Read the model definition and answer for the solid it produces. Units are mm, in the model's axes. A direction names the side the tool comes from. Give positions to 0.01 mm unless a question says otherwise; leave off trailing zeros. Write each loop counter-clockwise with the first axis right and the second up, starting at its lowest first coordinate (ties: lowest second). Pieces come first, ordered by that corner, then holes. Notation, with made-up numbers: (18, 11) -> (36, 11) arc R33 ccw to (36, 48) -> close; hole circle Ø2 at (-12.5, 84). An arc over 180 degrees is marked (long way). Put each result on its own line as item: value. Start each with the question number.
from build123d import *

# Parameters (mm, degrees)
F0_R     = 14.2875
F1_DEPTH = 25.4
F2_DEPTH = 25.4
F3_DEPTH = 50.8


with BuildPart() as f1:
    # F0 (on Front) → F1 (new body)
    with BuildSketch(Plane.XZ):
        with BuildLine():
            ThreePointArc((5.2887591577, -28.0813043068), (21.9961009946, -18.240125165), (28.575, 0))
            ThreePointArc((28.575, 0), (22.118144808, 18.0919400633), (5.6655830094, 28.0077095487))
            ThreePointArc((5.6655830094, 28.0077095487), (-28.5743551441, 0.1919716148), (5.2887591577, -28.0813043068))
        make_face()
        with BuildLine():
            ThreePointArc((-13.4703841816, 4.7625), (0, 14.2875), (13.4703841816, 4.7625))
            Line((13.4703841816, 4.7625), (22.225, 4.7625))
            Line((22.225, 4.7625), (22.225, -4.7625))
            Line((22.225, -4.7625), (13.4703841816, -4.7625))
            ThreePointArc((13.4703841816, -4.7625), (0, -14.2875), (-13.4703841816, -4.7625))
            Line((-13.4703841816, -4.7625), (-22.225, -4.7625))
            Line((-22.225, -4.7625), (-22.225, 4.7625))
            Line((-22.225, 4.7625), (-13.4703841816, 4.7625))
        make_face(mode=Mode.SUBTRACT)
        with BuildLine():
            ThreePointArc((73.025, 0), (66.3713381906, 14.464898875), (51.0582494002, 18.8253835536))
            ThreePointArc((51.0582494002, 18.8253835536), (34.9584276531, -1.1280408576), (53.304272269, -19.0381885775))
            ThreePointArc((53.304272269, -19.0381885775), (67.2061212058, -13.7054708652), (73.025, 0))
        make_face()
        with Locations((53.975, 0)):
            Circle(F0_R, mode=Mode.SUBTRACT)
        with BuildLine():
            ThreePointArc((5.6655830094, 28.0077095487), (22.118144808, 18.0919400633), (28.575, 0))
            ThreePointArc((28.575, 0), (21.9961009946, -18.240125165), (5.2887591577, -28.0813043068))
            Line((5.2887591577, -28.0813043068), (53.304272269, -19.0381885775))
            ThreePointArc((53.304272269, -19.0381885775), (34.9584276531, -1.1280408576), (51.0582494002, 18.8253835536))
            Line((51.0582494002, 18.8253835536), (5.6655830094, 28.0077095487))
        make_face()
        with BuildLine():
            ThreePointArc((-13.4703841816, -4.7625), (-14.2875, 0), (-13.4703841816, 4.7625))
            Line((-13.4703841816, 4.7625), (-22.225, 4.7625))
            Line((-22.225, 4.7625), (-22.225, -4.7625))
            Line((-22.225, -4.7625), (-13.4703841816, -4.7625))
        make_face()
    extrude(amount=F1_DEPTH)

    # F0 (on Front) → F2 (join)
    with BuildSketch(Plane.XZ):
        with BuildLine():
            ThreePointArc((5.6655830094, 28.0077095487), (22.118144808, 18.0919400633), (28.575, 0))
            ThreePointArc((28.575, 0), (21.9961009946, -18.240125165), (5.2887591577, -28.0813043068))
            Line((5.2887591577, -28.0813043068), (53.304272269, -19.0381885775))
            ThreePointArc((53.304272269, -19.0381885775), (34.9584276531, -1.1280408576), (51.0582494002, 18.8253835536))
            Line((51.0582494002, 18.8253835536), (5.6655830094, 28.0077095487))
        make_face()
        with BuildLine():
            Line((-13.4703841816, 4.7625), (13.4703841816, 4.7625))
            ThreePointArc((13.4703841816, 4.7625), (0, 14.2875), (-13.4703841816, 4.7625))
        make_face()
        with BuildLine():
            ThreePointArc((-13.4703841816, -4.7625), (0, -14.2875), (13.4703841816, -4.7625))
            Line((13.4703841816, -4.7625), (-13.4703841816, -4.7625))
        make_face()
    extrude(amount=F2_DEPTH)

    # F0 (on Front) → F3 (join)
    with BuildSketch(Plane.XZ):
        with BuildLine():
            ThreePointArc((5.2887591577, -28.0813043068), (21.9961009946, -18.240125165), (28.575, 0))
            ThreePointArc((28.575, 0), (22.118144808, 18.0919400633), (5.6655830094, 28.0077095487))
            ThreePointArc((5.6655830094, 28.0077095487), (-28.5743551441, 0.1919716148), (5.2887591577, -28.0813043068))
        make_face()
        with BuildLine():
            ThreePointArc((-13.4703841816, 4.7625), (0, 14.2875), (13.4703841816, 4.7625))
            Line((13.4703841816, 4.7625), (22.225, 4.7625))
            Line((22.225, 4.7625), (22.225, -4.7625))
            Line((22.225, -4.7625), (13.4703841816, -4.7625))
            ThreePointArc((13.4703841816, -4.7625), (0, -14.2875), (-13.4703841816, -4.7625))
            Line((-13.4703841816, -4.7625), (-22.225, -4.7625))
            Line((-22.225, -4.7625), (-22.225, 4.7625))
            Line((-22.225, 4.7625), (-13.4703841816, 4.7625))
        make_face(mode=Mode.SUBTRACT)
    extrude(amount=F3_DEPTH)


solid = f1.part
1) A cutting plane is placed at D-D on x = 66.5. Give the vertices of the cut face in (y, z), and give its area (3 significant figures).
2) A cutting plane is placed at A-A on x = 0. Give the vertices of the cut face in (y, z) (1 decimal).
3) Straight lines are drawn through the part: line 1 (X direction, y = -10, z = 2.5) (3 decimals); line 2 (Y direction, x = 33.5, z = 9); line 3 (Z direction, x = 21, y = -7). For each, find the intervals that lie inside material, in ascending order. Write a range as [from, to].
4) Each of these flat-tipped pins is pushed along its axis until it touches: pin 1 Ø7 at (x, z) = (-19.5, -2) entering from -Y; pin 2 Ø1 at (x, y) = (3, -26.5) entering from +Z; pin 3 Ø18 at (x, y) = (10, -27) entering from +Z; pin 4 Ø2 at (y, z) = (-30.5, -14) entering from -X. Where does it stop, or does it pass through?
5) For faces 4 (the face through (-7, -50.8, 13)), 5 (the face through (-14.287, -12.522, -0.068)), 6 (the face through (-18, -38, 4.762)), determine the directions among +Z, -Z, +X, -X, +Y, -Y from which every point of the face is accessible in a straight line to the end or side of a thin tool.
6) A cutting plane is placed at B-B on z = 9. Give the vertices of the cut face in (x, y).
7) For a pull along X with two mould halves and no side action, classify faces 1 (the face through (39, -25.4, -2)), 2 (the face through (8, -19, 4.762)), 3 (the face through (28.96, -12.522, -23.623)) as pulls with the +X half, pulls with the -X half, needs draft (parallel to the pull), parting line crosses it, or undercut.
Results found:
1. outline: (-25.4, -14.35) -> (0, -14.35) -> (0, -6.87) -> (-25.4, -6.87) -> close; (-25.4, 6.87) -> (0, 6.87) -> (0, 14.35) -> (-25.4, 14.35) -> close
1. area: 380 mm²
2. outline: (-50.8, -28.6) -> (0, -28.6) -> (0, -4.8) -> (-25.4, -4.8) -> (-25.4, -14.3) -> (-50.8, -14.3) -> close; (-50.8, 14.3) -> (-25.4, 14.3) -> (-25.4, 4.8) -> (0, 4.8) -> (0, 28.6) -> (-50.8, 28.6) -> close
3. line 1: x = [-28.465, -14.067], [22.225, 39.908], [68.042, 72.86]
3. line 2: y = [-25.4, 0]
3. line 3: z = [-25.12, -4.76], [4.76, 24.91]
4. pin 1: stops at y = -50.8
4. pin 2: stops at z = 28.47
4. pin 3: stops at z = 28.56
4. pin 4: stops at x = -25.45
5. face 4: +Z, -Z, +X, -X, -Y
5. face 5: +Y, -Y
5. face 6: -Y
6. outline: (-27.12, -50.8) -> (-11.1, -50.8) -> (-11.1, -25.4) -> (11.1, -25.4) -> (11.1, -50.8) -> (27.12, -50.8) -> (27.12, -25.4) -> (42.88, -25.4) -> (42.88, 0) -> (-27.12, 0) -> close; (65.07, -25.4) -> (70.76, -25.4) -> (70.76, 0) -> (65.07, 0) -> close
7. face 1: needs draft
7. face 2: undercut
7. face 3: pulls with the +X half
